```python
from build123d import *

# Parameters (mm, degrees)
BOSS_EXTRUDE1_DEPTH                             = 28.8
SKETCH2_W                                       = 2.75
SKETCH2_H                                       = 3.75
CUT_EXTRUDE1_DEPTH                              = 3.75
CUT_EXTRUDE2_START                              = -2
CUT_EXTRUDE2_DEPTH                              = 53.6
SKETCH4_W                                       = 53.6
SKETCH4_H                                       = 54.504926328
CUT_EXTRUDE3_DEPTH                              = 8
CSK_FOR_M3_FLAT_HEAD_MACHINE_SCREW1_D           = 3.4
CSK_FOR_M3_FLAT_HEAD_MACHINE_SCREW1_DEPTH       = 7.874
CSK_FOR_M3_FLAT_HEAD_MACHINE_SCREW1_CSINK_D     = 6.3
CSK_FOR_M3_FLAT_HEAD_MACHINE_SCREW1_CSINK_ANGLE = 90
CSK_FOR_M3_FLAT_HEAD_MACHINE_SCREW1_TIP         = 1.021463052
CUT_EXTRUDE4_DEPTH                              = 45.893652113


with BuildPart() as part:
    # Sketch1 → Boss-Extrude1 (new, symmetric)
    with BuildSketch(Plane(origin=(0, 0, 0), x_dir=(0, 0, -1), z_dir=(1, 0, 0))):
        with BuildLine():
            Line((0, 0), (31, 0))
            Line((31, 0), (31, 11.5))
            ThreePointArc((31, 11.5), (29.974873734, 13.974873734), (27.5, 15))
            Line((27.5, 15), (0, 15))
            Line((0, 15), (0, 0))
        make_face()
    boss_extrude1 = extrude(amount=BOSS_EXTRUDE1_DEPTH, both=True)

    # Mirror1: Boss-Extrude1 across plane
    add(boss_extrude1.mirror(Plane(origin=(28.8, 15, 0), x_dir=(1, 0, 0), z_dir=(0, 0, -1))))

    # Sketch2 → Cut-Extrude1 (cut)
    with BuildSketch(Plane(origin=(28.8, 0, 0), x_dir=(0, 0, -1), z_dir=(1, 0, 0))):
        with Locations((-16.8750001, 1.875)):
            Rectangle(SKETCH2_W, SKETCH2_H)
        with Locations((-13.1250001, 1.875)):
            Rectangle(SKETCH2_W, SKETCH2_H)
    extrude(amount=-CUT_EXTRUDE1_DEPTH, mode=Mode.SUBTRACT)

    # Sketch3 → Cut-Extrude2 (cut)
    with BuildSketch(Plane(origin=(28.8, 0, 0), x_dir=(0, 0, -1), z_dir=(1, 0, 0)).offset(CUT_EXTRUDE2_START)):
        with BuildLine():
            Line((-30.270000062, 9.160000031), (-30.270000062, 2))
            Line((-30.270000062, 2), (-15.95, 2))
            Line((-15.95, 2), (-15.95, 9.160000031))
            ThreePointArc((-15.95, 9.160000031), (-23.110000031, 16.320000062), (-30.270000062, 9.160000031))
        make_face()
        with BuildLine():
            Line((-14.863333375, 9.160000031), (-14.863333375, 2))
            Line((-14.863333375, 2), (-0.543333313, 2))
            Line((-0.543333313, 2), (-0.543333313, 9.160000031))
            ThreePointArc((-0.543333313, 9.160000031), (-7.703333344, 16.320000062), (-14.863333375, 9.160000031))
        make_face()
    cut_extrude2 = extrude(amount=-CUT_EXTRUDE2_DEPTH, mode=Mode.SUBTRACT)

    # Mirror2: Cut-Extrude2 across plane
    add(cut_extrude2.mirror(Plane.XY), mode=Mode.SUBTRACT)

    # Sketch4 → Cut-Extrude3 (cut)
    with BuildSketch(Plane(origin=(0, 15, 0), x_dir=(1, 0, 0), z_dir=(0, 1, 0))):
        Rectangle(SKETCH4_W, SKETCH4_H)
    extrude(amount=-CUT_EXTRUDE3_DEPTH, mode=Mode.SUBTRACT)

    # CSK for M3 Flat Head Machine Screw1
    with Locations(Plane(origin=(0, 2, -22.5), x_dir=(0, 0, 1), z_dir=(0, 1, 0))):
        with Locations((0, 0), (15, 0), (30, 0), (45, 0)):
            CounterSinkHole(CSK_FOR_M3_FLAT_HEAD_MACHINE_SCREW1_D / 2, CSK_FOR_M3_FLAT_HEAD_MACHINE_SCREW1_CSINK_D / 2, depth=CSK_FOR_M3_FLAT_HEAD_MACHINE_SCREW1_DEPTH, counter_sink_angle=CSK_FOR_M3_FLAT_HEAD_MACHINE_SCREW1_CSINK_ANGLE)
            with Locations((0, 0, -(CSK_FOR_M3_FLAT_HEAD_MACHINE_SCREW1_DEPTH + CSK_FOR_M3_FLAT_HEAD_MACHINE_SCREW1_TIP / 2))):  # 118° drill point
                Cone(0, CSK_FOR_M3_FLAT_HEAD_MACHINE_SCREW1_D / 2, CSK_FOR_M3_FLAT_HEAD_MACHINE_SCREW1_TIP, mode=Mode.SUBTRACT)

    # Sketch7 → Cut-Extrude4 (cut, symmetric)
    with BuildSketch(Plane.XY):
        with BuildLine():
            Line((-26.8, 15), (-26.8, 7.5))
            Line((-26.8, 7.5), (-25.551032793, 7.5))
            ThreePointArc((-25.551032793, 7.5), (-24.233583531, 7.995231765), (-23.568576992, 9.23567256))
            Line((-23.568576992, 9.23567256), (-23.031423008, 13.26432744))
            ThreePointArc((-23.031423008, 13.26432744), (-22.366416469, 14.504768235), (-21.048967207, 15))
            Line((-21.048967207, 15), (-22.8, 15))
            Line((-22.8, 15), (-26.8, 15))
        make_face()
        with BuildLine():
            Line((-9.568576992, 13.26432744), (-9.031423008, 9.23567256))
            ThreePointArc((-9.031423008, 9.23567256), (-8.366416469, 7.995231765), (-7.048967207, 7.5))
            Line((-7.048967207, 7.5), (0, 7.5))
            Line((0, 7.5), (0, 15))
            Line((0, 15), (-9.8, 15))
            Line((-9.8, 15), (-11.551032793, 15))
            ThreePointArc((-11.551032793, 15), (-10.233583531, 14.504768235), (-9.568576992, 13.26432744))
        make_face()
    cut_extrude4 = extrude(amount=CUT_EXTRUDE4_DEPTH, both=True, mode=Mode.SUBTRACT)

    # Mirror3: Cut-Extrude4 across plane
    add(cut_extrude4.mirror(Plane(origin=(0, 0, 0), x_dir=(0, 0, 1), z_dir=(1, 0, 0))), mode=Mode.SUBTRACT)


solid = part.part
```
Design review of the part built by this model. Coordinates are the model's own, in mm. A direction names the side the tool comes from. Coordinates: 2 decimals unless noted, no trailing zeros. Write each loop counter-clockwise with the first axis right and the second up, starting at its lowest first coordinate (ties: lowest second). Pieces come first, ordered by that corner, then holes. Notation, with made-up numbers: M -4.5,-33.5 L 38.5,-33.5 A30 cw 38.5,1.5 Z; hole C -39.5,12.5 d8. An arc over 180 degrees is marked long. Answer as a JSON object with one key per item and string values.
Item 1: Add section A-A, the plane y = 2.75. Give the boundary of the cut face in (x, z), and give its area (3 significant figures).
Outcome:
{"outline": "M -28.8,-31 L 28.8,-31 L 28.8,11.75 L 26.8,11.75 L 26.8,0.54 L -26.8,0.54 L -26.8,14.86 L 26.8,14.86 L 26.8,14.5 L 28.8,14.5 L 28.8,15.5 L 25.05,15.5 L 25.05,15.95 L -26.8,15.95 L -26.8,30.27 L 26.8,30.27 L 26.8,18.25 L 28.8,18.25 L 28.8,31 L -28.8,31 Z; hole M -26.8,-30.27 L 26.8,-30.27 L 26.8,-15.95 L -26.8,-15.95 Z; hole M -26.8,-14.86 L 26.8,-14.86 L 26.8,-0.54 L -26.8,-0.54 Z", "area": "489 mm²"}
Item 2: Add section D-D, the plane z = -17.5. Give the boundary of the cut face in (x, y), and give its area (3 significant figures).
Outcome:
{"outline": "M -28.8,0 L 28.8,0 L 28.8,15 L 26.8,15 L 26.8,2 L -26.8,2 L -26.8,15 L -28.8,15 Z", "area": "167 mm²"}
Item 3: Add section C-C, the plane y = 10.25. Give the boundary of the cut face in (x, z).
Outcome:
{"outline": "M -28.8,-31 L -26.8,-31 L -26.8,31 L -28.8,31 Z; M -23.43,-31 L -9.17,-31 L -9.17,-30.19 L -23.43,-30.19 Z; M -23.43,30.19 L -9.17,30.19 L -9.17,31 L -23.43,31 Z; M 9.17,-31 L 23.43,-31 L 23.43,-30.19 L 9.17,-30.19 Z; M 9.17,30.19 L 23.43,30.19 L 23.43,31 L 9.17,31 Z; M 26.8,-31 L 28.8,-31 L 28.8,31 L 26.8,31 Z"}
Item 4: Insertion check: pin 1 Ø0.6 at (x, z) = (-2.5, -30.5) entering from +Y; pin 2 Ø8 at (x, z) = (-17.5, 5.5) entering from +Y; pin 3 Ø2 at (x, z) = (-13.5, -17) entering from -Y; pin 4 Ø0.8 at (y, z) = (1, 16.5) entering from +X. Each pin has a flat end and moves straight along its axis. Give the tip position at first contact, or say it passes through.
Outcome:
{"pin 1": "y = 7.5", "pin 2": "y = 2", "pin 3": "y = 0", "pin 4": "x = 25.05"}
Item 5: Wall thickness on probe 1 along Z at (x, y) = (18.5, 5.75); probe 2 along X at (y, z) = (9.75, 15); probe 3 along Z at (x, y) = (0, 0.25): over which ranges is each line inside the solid? List them lowest first.
Outcome:
{"probe 1": "-31 to -30.27, -15.95 to -14.86, -0.54 to 0.54, 14.86 to 15.95, 30.27 to 31", "probe 2": "-28.8 to -26.8, 26.8 to 28.8", "probe 3": "-31 to -24.2, -20.8 to -9.2, -5.8 to 5.8, 9.2 to 20.8, 24.2 to 31"}
Item 6: Draft analysis for pull direction Z (two halves, no side actions). For faces 1 (the cylindrical face through (27.81, 13.95, -30)), 2 (the cylindrical face through (-16.2, 12.49, 29.45)), 3 (the flat face through (0, 2, -11)), 4 (the flat face through (-28, 15, 0)), state which applies: pulls with the +Z half, pulls with the -Z half, needs draft (parallel to the pull), parting line crosses it, or undercut.
Outcome:
{"face 1": "pulls with the -Z half", "face 2": "undercut", "face 3": "undercut", "face 4": "needs draft"}
Item 7: Add section B-B, the plane z = 7.5. Give the boundary of the cut face in (x, y), and give its area (3 significant figures).
Outcome:
{"outline": "M -28.8,0 L -1.7,0 L -1.7,0.55 L -3.15,2 L -26.8,2 L -26.8,15 L -28.8,15 Z; M 1.7,0 L 28.8,0 L 28.8,15 L 26.8,15 L 26.8,2 L 3.15,2 L 1.7,0.55 Z", "area": "158 mm²"}
Item 8: Machinability: for faces 5 (the cylindrical face through (8.381, 8.009, -30.63)), 6 (the cylindrical face through (-1.03, 0.27, 8.85)), 7 (the flat face through (0, 4, 0.543)), which of the approach directions +Z, -Z, +X, -X, +Y, -Y give a long, thin tool a straight path to every point of the face, cutting with its end or side? Answer none if there is none.
Outcome:
{"face 5": "+Z, -Z, +Y", "face 6": "+Y, -Y", "face 7": "+Y"}
